Here's how the part is built. I have some questions about the finished solid (model axes, mm). Coordinates: 2 decimals unless noted, no trailing zeros. Write each loop counter-clockwise with the first axis right and the second up, starting at its lowest first coordinate (ties: lowest second). Pieces come first, ordered by that corner, then holes.
Item 1: I want a section at D-D (x = 33). Please give me the cut outline in (y, z).
Item 2: I want a section at C-C (y = 7.75). Count the separate pieces of the cut face and the enclosed holes in it, and give its area (3 significant figures).
Item 3: I'm going to push flat-ended pins straight in: P1, Ø3, axis at y = 2.5, z = 39, coming from the -X side; P2, Ø9.5, axis at x = 31.75, z = 71.6, coming from the -Y side. Where does each tip first touch, or does it pass through?
Item 4: If we mould it in two halves opening along X, with no side actions, what happens to faces 1 (the face through (0.55, 4.93, 49.997)), 2 (the face through (47.18, 4.93, 77.71)), 3 (the face through (1, 0, 62))? For each: pulls with the +X half, pulls with the -X half, needs draft (parallel to the pull), parting line crosses it, or undercut.
Item 5: I want a section at B-B (z = 69). Please give me the cut outline in (x, y).
Item 6: I want a section at A-A (x = -31.75). Please give me the cut outline in (y, z).
Item 7: Please list where these lines run through material, in increasing order: line 1 (Z direction, x = 41.25, y = 5); line 2 (X direction, y = 6.75, z = 71.6); line 3 (X direction, y = 3.5, z = 41.25).
Solid Edge part; units mm, degrees
sketch "Sketch1" plane through (0, 0, 0) normal (0, -1, 0) x (1, 0, 0)
  arc A0 (-35.3553, 35.3553) -> (35.3553, 35.3553) centre (0, 0) cw
  arc A1 (35.3553, 35.3553) -> (49.5863, 41.25) centre (41.25, 41.25) ccw
  line L0 (49.5863, 41.25) -> (49.5863, 71.6)
  arc A2 (49.5863, 71.6) -> (31.75, 89.4363) centre (31.75, 71.6) ccw
  line L1 (-31.75, 89.4363) -> (31.75, 89.4363)
  arc A3 (-49.5863, 71.6) -> (-31.75, 89.4363) centre (-31.75, 71.6) cw
  line L2 (-49.5863, 41.25) -> (-49.5863, 71.6)
  arc A4 (-35.3553, 35.3553) -> (-49.5863, 41.25) centre (-41.25, 41.25) cw
  dimension "D1" = 49.5863
  dimension "D2" = 49.5863
extrude "Protrusion1" add sketch "Sketch1" against normal blind 10
thread "Thread1" [suppressed]
thread "Thread2" [suppressed]
hole "Hole_1" at (-31.75, 0, 71.6) direction (0, 1, 0) diameter 8.4 end up to next
hole "Hole1" at (31.75, 0, 71.6) direction (0, 1, 0) diameter 8.4 end up to next
sketch "Sketch2" plane through (0, 0, 61.425) normal (0, -1, 0) x (1, 0, 0)
  line L0 (-83.4503, 18.575) -> (83.4503, 18.575)
  dimension "D1" = 83.4503
extrude "ExtrudedCutout_1" cut sketch "Sketch2" against normal blind 30.8448 and the other way blind 163.4824 material side at (0, 0, 80.05)
fillet "Round_1" radius 8 1 edges at (47.4845, 5, 80)
fillet "Round_2" radius 10 1 edges at (-47.4845, 5, 80)
hole "Hole_3" at (-41.25, 0, 41.25) direction (0, 1, 0) diameter 8.376 end up to next thread major 10 thread length 2
hole "Hole2" at (41.25, 0, 41.25) direction (0, 1, 0) diameter 8.376 end up to next thread major 10 thread length 2
properties material "Iron, grey cast type 40"
Answer:
1. outline: (0, 37.56) - (10, 37.56) - (10, 67.59) - (0, 67.59) - close; (0, 75.61) - (10, 75.61) - (10, 80) - (0, 80) - close
2. separate pieces: 1
2. enclosed holes: 4
2. area: 3,490 mm2
3. P1: stops at x = -49.55
3. P2: stops at y = 0
4. face 1: undercut
4. face 2: pulls with the +X half
4. face 3: needs draft
5. outline: (-49.59, 0) - (-35.05, 0) - (-35.05, 10) - (-49.59, 10) - close; (-28.45, 0) - (28.45, 0) - (28.45, 10) - (-28.45, 10) - close; (35.05, 0) - (49.59, 0) - (49.59, 10) - (35.05, 10) - close
6. outline: (0, 38.63) - (10, 38.63) - (10, 67.4) - (0, 67.4) - close; (0, 75.8) - (10, 75.8) - (10, 80) - (0, 80) - close
7. line 1: z = 32.91 to 37.06, 45.44 to 80
7. line 2: x = -49.46 to -35.95, -27.55 to 27.55, 35.95 to 49.59
7. line 3: x = -49.59 to -45.44, -37.06 to -28.26, 28.26 to 37.06, 45.44 to 49.59
